Read the model definition and answer for the solid it produces. Units are mm, in the model's axes. A direction names the side the tool comes from. Give positions to 0.01 mm unless a question says otherwise; leave off trailing zeros. Loops run counter-clockwise (first coordinate to the right, second up) from the corner with the lowest first, then second, coordinate; pieces in that order, holes last. Notation, with made-up numbers: (8, 41) -> (12, 41) arc R13 ccw to (12, 54) -> close; hole circle Ø1 at (68.5, -39). An arc over 180 degrees is marked (long way). Write each question's results on one line, items separated by ' | '. Start each with the question number.
Item 1: Find the intervals of material crossed by line 1 (Z direction, x = -0.7, y = -1.5); line 2 (Z direction, x = -0.4, y = 0.45); line 3 (Y direction, x = -0.05, z = -6.25), in increasing order.
Item 2: Which of the six approach directions +Z, -Z, +X, -X, +Y, -Y give full straight-line access (tool end or side, diameter ignored) to faces 4 (the flat face through (-0.63, 1.08, -11.36)), 5 (the cylindrical face through (-1.5, -0.07, -5.03))?
Item 3: Determine the mould class of faces 1 (the flat face through (-1.25, 0, -11)), 2 (the cylindrical face through (-0.29, -2.23, -10.99)), 3 (the flat face through (0, 0, 0)) for opening direction X: +X half, -X half, draft (parallel to the pull), parting line (faces both ways), or undercut.
Item 4: Section B-B on z = -4.5 is taken. Write down the section's boundary in (x, y).
Item 5: Section A-A on y = 0 is taken. Write down the section's boundary in (x, z).
Item 6: Each of these flat-tipped pins is pushed along its axis until it touches: P1, Ø1.5, axis at y = -0.5, z = -8.5, coming from the +X side; P2, Ø0.6, axis at x = 0, y = 0, coming from the -Z side; P3, Ø1, axis at x = -1.5, z = -8.5, coming from the +Y side. Where does it stop, or does it pass through?
```python
from build123d import *

# Parameters (mm, degrees)
CUT_EXTRUDE1_DEPTH = 1.5
CHAMFER1_SIZE      = 0.2


with BuildPart() as part:
    # Sketch1 → Revolve1 (revolve)
    with BuildSketch(Plane(origin=(0, 0, 0), x_dir=(1, 0, 0), z_dir=(0, 1, 0))):
        with BuildLine():
            Line((0, 12), (2.05, 12))
            ThreePointArc((2.05, 12), (2.191421356, 11.941421356), (2.25, 11.8))
            Line((2.25, 11.8), (2.25, 10.2))
            ThreePointArc((2.25, 10.2), (2.191421356, 10.058578644), (2.05, 10))
            Line((2.05, 10), (1.5, 10))
            Line((1.5, 10), (1.5, 0.2))
            Line((1.5, 0.2), (1.3, 0))
            Line((1.3, 0), (0, 0))
            Line((0, 0), (0, 12))
        make_face()
    revolve(axis=Axis((0, 0, 0), (0, 0, -1)))

    # Sketch2 → Cut-Extrude1 (cut)
    with BuildSketch(Plane(origin=(0, 0, -12), x_dir=(-1, 0, 0), z_dir=(0, 0, -1))):
        Polygon((1.25, 0.721687836), (0, 1.443375673), (-1.25, 0.721687836), (-1.25, -0.721687836), (0, -1.443375673), (1.25, -0.721687836), align=None)
    extrude(amount=-CUT_EXTRUDE1_DEPTH, mode=Mode.SUBTRACT)

    # Chamfer1
    chamfer1_edges = [part.edges().sort_by_distance(p)[0] for p in [
        (-1.25, 0, -10.5),
        (-0.625, -1.082531755, -10.5),
        (0.625, -1.082531755, -10.5),
        (1.25, 0, -10.5),
        (0.625, 1.082531755, -10.5),
        (-0.625, 1.082531755, -10.5),
    ]]
    chamfer(chamfer1_edges, length=CHAMFER1_SIZE)


solid = part.part
```
Findings:
1) line 1: -12 to -10 | line 2: -10.5 to 0 | line 3: -1.5 to 1.5
2) face 4: -Z | face 5: +Z
3) face 1: undercut | face 2: parting line | face 3: draft
4) outline: circle Ø3 at (0, 0)
5) outline: (-2.25, -11.8) arc R0.2 ccw to (-2.05, -12) -> (-1.25, -12) -> (-1.25, -10.7) -> (-1.05, -10.5) -> (1.05, -10.5) -> (1.25, -10.7) -> (1.25, -12) -> (2.05, -12) arc R0.2 ccw to (2.25, -11.8) -> (2.25, -10.2) arc R0.2 ccw to (2.05, -10) -> (1.5, -10) -> (1.5, -0.2) -> (1.3, 0) -> (-1.3, 0) -> (-1.5, -0.2) -> (-1.5, -10) -> (-2.05, -10) arc R0.2 ccw to (-2.25, -10.2) -> close
6) P1: x = 1.5 | P2: z = -10.5 | P3: y = 1.12
